Answer from the drawing. Dimensions are ordinates in mm from the lowest x, y and z of the part. Give positions to 0.01 mm unless a question says otherwise; leave off trailing zeros. Order: outer loops, then holes, each group sorted by start corner. A loop starts at its lowest first (then second) coordinate and runs counter-clockwise, first axis right, second up. Notation, with made-up numbers: (3, 65.5) - (23, 65.5) arc R8 cw to (23, 70.5) - close; hole circle Ø6 at (55.5, 37.5). An arc over 180 degrees is marked (long way). Write each question's results on one line, items separated by ' | '.
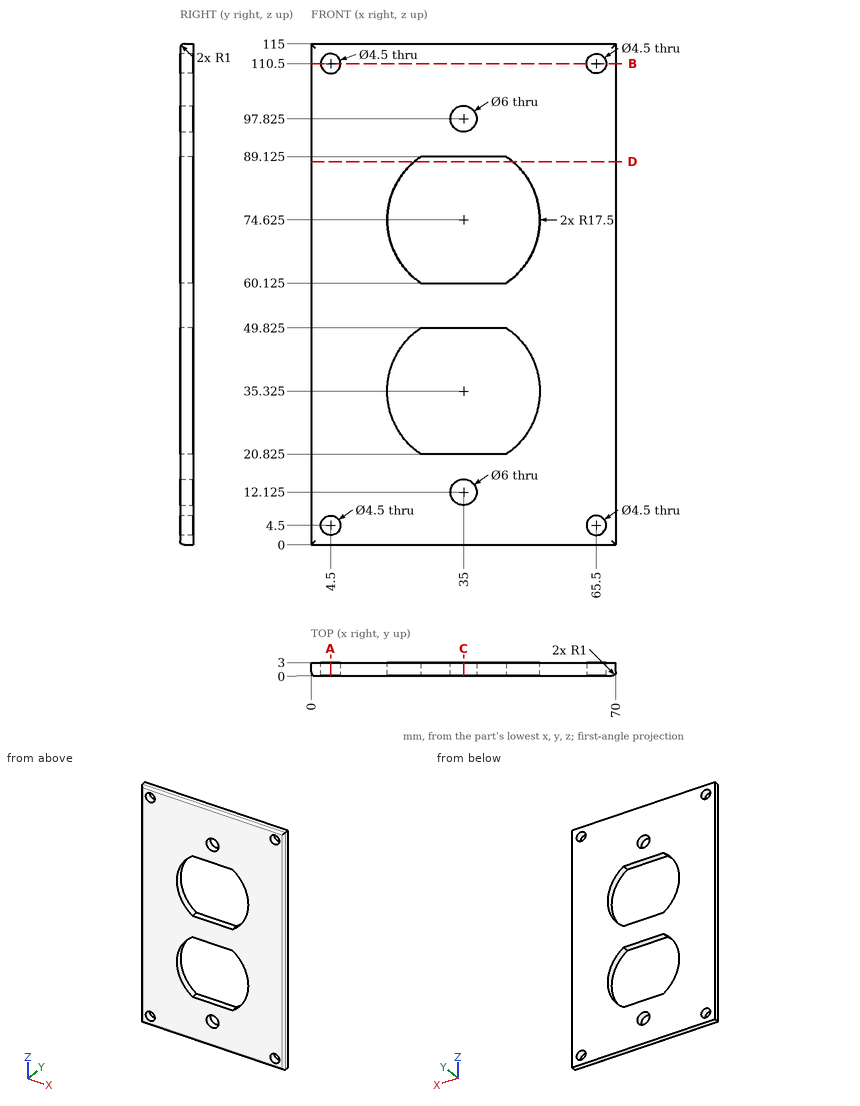
1. A cutting plane is placed at A-A, the plane x = 4.5. Write down the section's boundary in (y, z).
Answer list:
outline: (0, 1) arc R1 ccw to (1, 0) - (3, 0) - (3, 2.25) - (0, 2.25) - close; (0, 6.75) - (3, 6.75) - (3, 108.25) - (0, 108.25) - close; (0, 112.75) - (3, 112.75) - (3, 115) - (1, 115) arc R1 ccw to (0, 114) - close
2. A cutting plane is placed at D-D, the plane z = 88. Write down the section's boundary in (x, y), then the cut area to 3 significant figures.
Answer list:
outline: (0, 1) arc R1 ccw to (1, 0) - (23.71, 0) - (23.71, 3) - (0, 3) - close; (46.29, 0) - (69, 0) arc R1 ccw to (70, 1) - (70, 3) - (46.29, 3) - close | area: 142 mm^2
3. A cutting plane is placed at C-C, the plane x = 35. Write down the section's boundary in (y, z) (3 decimals).
Answer list:
outline: (0, 1) arc R1 ccw to (1, 0) - (3, 0) - (3, 9.125) - (0, 9.125) - close; (0, 15.125) - (3, 15.125) - (3, 20.825) - (0, 20.825) - close; (0, 49.825) - (3, 49.825) - (3, 60.125) - (0, 60.125) - close; (0, 89.125) - (3, 89.125) - (3, 94.825) - (0, 94.825) - close; (0, 100.825) - (3, 100.825) - (3, 115) - (1, 115) arc R1 ccw to (0, 114) - close
4. Straight lines are drawn through the part: line 1 (Z direction, x = 35, y = 1.1) (3 decimals); line 2 (Z direction, x = 65.5, y = 1.6); line 3 (Z direction, x = 41.5, y = 2) (3 decimals). For each, find the intervals that lie inside material, in ascending order. Write a range as [from, to].
Answer list:
line 1: [0, 9.125], [15.125, 20.825], [49.825, 60.125], [89.125, 94.825], [100.825, 115] | line 2: [0, 2.25], [6.75, 108.25], [112.75, 115] | line 3: [0, 20.825], [49.825, 60.125], [89.125, 115]
5. A cutting plane is placed at B-B, the plane z = 110.5. Write down the section's boundary in (x, y), then the cut area to 3 significant figures.
Answer list:
outline: (0, 1) arc R1 ccw to (1, 0) - (2.25, 0) - (2.25, 3) - (0, 3) - close; (6.75, 0) - (63.25, 0) - (63.25, 3) - (6.75, 3) - close; (67.75, 0) - (69, 0) arc R1 ccw to (70, 1) - (70, 3) - (67.75, 3) - close | area: 183 mm^2
